Check sheet for the drawn part. Datum: minimum x, y, z corner. Units: mm. Coordinates: 2 decimals unless noted, no trailing zeros. Write each loop counter-clockwise with the first axis right and the second up, starting at its lowest first coordinate (ties: lowest second). Pieces come first, ordered by that corner, then holes. Notation, with made-up numbers: (12, 38) -> (38, 38) arc R18 cw to (38, 71) -> close; hole circle Ø10 at (46.5, 10). An arc over 180 degrees is marked (long way). Answer in a Markdown table with one row per item.
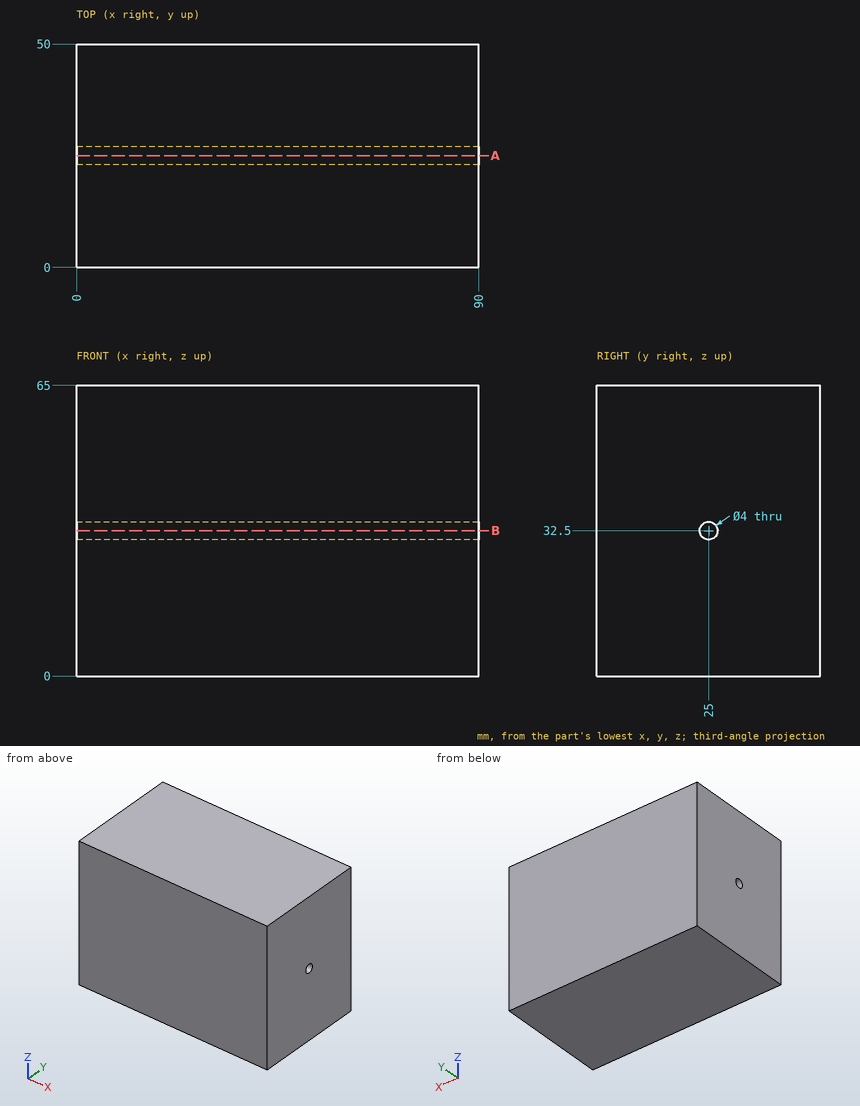
1. Sectioned sample at A-A, the plane y = 25. Record the cut outline in (x, z), and give its area (3 significant figures).
Findings below:
| item | result |
|---|---|
| outline | (0, 0) -> (90, 0) -> (90, 30.5) -> (0, 30.5) -> close; (0, 34.5) -> (90, 34.5) -> (90, 65) -> (0, 65) -> close |
| area | 5,490 mm² |
2. Go/stop test with flat-tipped pins: pin 1 (3 mm diameter, centred on y = 25, z = 32.5, fed in from -X); pin 2 (8 mm diameter, centred on x = 56, z = 50, fed in from -Y). Record where each tip stops, or that it passes through.
Findings below:
| item | result |
|---|---|
| pin 1 | passes through |
| pin 2 | stops at y = 0 |
3. Sectioned sample at B-B, the plane z = 32.5. Record the cut outline in (x, y), and give its area (3 significant figures).
Findings below:
| item | result |
|---|---|
| outline | (0, 0) -> (90, 0) -> (90, 23) -> (0, 23) -> close; (0, 27) -> (90, 27) -> (90, 50) -> (0, 50) -> close |
| area | 4,140 mm² |
4. Material ranges on probe 1 along Y at (x, z) = (56.5, 32.5); probe 2 along Y at (x, z) = (29, 32); probe 3 along Z at (x, y) = (23, 26), recorded low to high. Write a range as from..to.
Findings below:
| item | result |
|---|---|
| probe 1 | y = 0..23, 27..50 |
| probe 2 | y = 0..23.06, 26.94..50 |
| probe 3 | z = 0..30.77, 34.23..65 |
